The listing builds one solid part. Answer for the finished solid, in the listing's coordinates (mm). A direction names the side the tool comes from. Coordinates: 2 decimals unless noted, no trailing zeros. Order: outer loops, then holes, each group sorted by start corner. A loop starts at its lowest first (then second) coordinate and runs counter-clockwise, first axis right, second up. Notation, with made-up numbers: (-1, 8) -> (16, 8) arc R17 cw to (16, 18) -> close; hole circle Ø11 at (35, 17). An arc over 180 degrees is marked (long way). One line per question, with ' | ' between items.
from build123d import *

# Parameters (mm, degrees)
F1_DEPTH = 453


with BuildPart() as f1:
    # F0 (on Right) → F1 (new body)
    with BuildSketch(Plane.YZ):
        with BuildLine():
            Line((-252, 0), (-169.264911, 0))
            Line((-169.264911, 0), (-169.264911, 35.794733))
            Line((-169.264911, 35.794733), (-253.264911, 7.794733))
            ThreePointArc((-253.264911, 7.794733), (-255.94835, 3.359271), (-252, 0))
        make_face()
        Polygon((-252, 4), (-173.264911, 30.24503), (-173.264911, 4), align=None, mode=Mode.SUBTRACT)
    extrude(amount=F1_DEPTH)


solid = f1.part
Item 1: Determine the mould class of faces 3 (the face through (223.33, -255.96, 3.44)), 4 (the face through (223, -213, 17)), 5 (the face through (223, -212, 4)), 6 (the face through (0, -210, 3)) for opening direction Z: pulls with the +Z half, pulls with the -Z half, needs draft (parallel to the pull), parting line crosses it, or undercut.
Computed values:
face 3: parting line crosses it | face 4: undercut | face 5: undercut | face 6: needs draft
Item 2: Each of these flat-tipped pins is pushed along its axis until it touches: pin 1 Ø1.5 at (y, z) = (-185.5, 5.5) entering from -X; pin 2 Ø23.5 at (x, y) = (318, -219.5) entering from +Z; pin 3 Ø8 at (x, y) = (132.5, -204.5) entering from +Z; pin 4 Ø6 at (x, y) = (93.5, -247.5) entering from +Z. Where does it stop, or does it pass through?
Computed values:
pin 1: passes through | pin 2: stops at z = 22.97 | pin 3: stops at z = 25.38 | pin 4: stops at z = 10.72
Item 3: Find the intervals of material crossed by L1, parallel to Z at x = 132.5, y = -179; L2, parallel to Z at x = 56, y = -227; L3, parallel to Z at x = 387.5, y = -173, in increasing order.
Computed values:
L1: z = 0 to 4, 28.33 to 32.55 | L2: z = 0 to 4, 12.33 to 16.55 | L3: z = 0 to 34.55
Item 4: For faces 1 (the face through (223, -173.265, 17)), 2 (the face through (223, -211, 0)), determine the directions among +Z, -Z, +X, -X, +Y, -Y from which every point of the face is accessible in a straight line to the end or side of a thin tool.
Computed values:
face 1: +X, -X | face 2: -Z, +X, -X, +Y, -Y
Item 5: Section B-B, the plane z = 24 is taken. Give the vertices of the cut face in (x, y), plus the area to 3 significant figures.
Computed values:
outline: (0, -204.65) -> (453, -204.65) -> (453, -192) -> (0, -192) -> close; (0, -173.26) -> (453, -173.26) -> (453, -169.26) -> (0, -169.26) -> close | area: 7,540 mm^2
Item 6: Section A-A, the plane x = 343 is taken. Give the vertices of the cut face in (y, z).
Computed values:
outline: (-253.26, 7.79) arc R4 ccw to (-252, 0) -> (-169.26, 0) -> (-169.26, 35.79) -> close; hole (-252, 4) -> (-173.26, 4) -> (-173.26, 30.25) -> close
Item 7: Section C-C, the plane y = -184 is taken. Give the vertices of the cut face in (x, z).
Computed values:
outline: (0, 0) -> (453, 0) -> (453, 4) -> (0, 4) -> close; (0, 26.67) -> (453, 26.67) -> (453, 30.88) -> (0, 30.88) -> close
